Verification items for the finished model (mm, model axes). A direction names the side the tool comes from. Give positions to 0.01 mm unless a question says otherwise; leave off trailing zeros. Order: outer loops, then holes, each group sorted by start corner. A loop starts at its lowest first (then second) coordinate and runs counter-clockwise, first axis right, second up.
from build123d import *

# Parameters (mm, degrees)
SKETCH1_R           = 21.05
BOSS_EXTRUDE1_DEPTH = 10.93
SKETCH2_R           = 15.65
BOSS_EXTRUDE2_DEPTH = 0.07
SKETCH3_W           = 7.03
SKETCH3_H           = 2.225
SKETCH5_R           = 12.545
BOSS_EXTRUDE3_DEPTH = 7.14
SKETCH6_R           = 4
CUT_EXTRUDE1_DEPTH  = 19.14


with BuildPart() as part:
    # Sketch1 → Boss-Extrude1 (new body)
    with BuildSketch(Plane(origin=(0, 0, 0), x_dir=(0, 0, -1), z_dir=(1, 0, 0))):
        Circle(SKETCH1_R)
    extrude(amount=BOSS_EXTRUDE1_DEPTH)

    # Sketch2 → Boss-Extrude2 (add)
    with BuildSketch(Plane(origin=(10.93, 0, 0), x_dir=(0, 0, -1), z_dir=(1, 0, 0))):
        Circle(SKETCH2_R)
    extrude(amount=BOSS_EXTRUDE2_DEPTH)

    # Mirror1: part across plane


with BuildPart() as part_1:
    add(part.part)
    add(part.part.mirror(Plane(origin=(5.465, 0, 0), x_dir=(0, 0, 1), z_dir=(1, 0, 0))))

    # Sketch3 → Cut-Revolve1 (revolve, cut)
    with BuildSketch(Plane.XY):
        with Locations((5.465, 19.9375)):
            Rectangle(SKETCH3_W, SKETCH3_H)
    revolve(axis=Axis((0, 0, 0), (1, 0, 0)), mode=Mode.SUBTRACT)

    # Sketch5 → Boss-Extrude3 (add)
    with BuildSketch(Plane(origin=(10.93, 0, 0), x_dir=(0, 0, -1), z_dir=(1, 0, 0))):
        Circle(SKETCH5_R)
    extrude(amount=BOSS_EXTRUDE3_DEPTH)

    # Sketch6 → Cut-Extrude1 (cut, through all)
    with BuildSketch(Plane(origin=(18.07, 0, 0), x_dir=(0, 0, -1), z_dir=(1, 0, 0))):
        Circle(SKETCH6_R)
    extrude(amount=-CUT_EXTRUDE1_DEPTH, mode=Mode.SUBTRACT)


solid = part_1.part
(1) Section check D-D, the plane z = -17.5. Enter the section's corners in (x, y).
Solved:
outline: (0, -11.7) - (1.95, -11.7) - (1.95, -6.94) - (8.98, -6.94) - (8.98, -11.7) - (10.93, -11.7) - (10.93, 11.7) - (8.98, 11.7) - (8.98, 6.94) - (1.95, 6.94) - (1.95, 11.7) - (0, 11.7) - close
(2) Release check for a two-part mould opening along X. For faces 4 (the flat face through (8.98, 16, -11)), 5 (the cylindrical face through (14.49, 12.44, 1.63)), 6 (the flat face through (18.07, 3, 3)) record: pulls with the +X half, pulls with the -X half, needs draft (parallel to the pull), parting line crosses it, or undercut.
Solved:
face 4: undercut
face 5: needs draft
face 6: pulls with the +X half
(3) Set-up check for faces 1 (the flat face through (1.95, 16, -11)), 2 (the flat face through (0, 16, 0)), 3 (the flat face through (11, 5, 12)): record each of +Z, -Z, +X, -X, +Y, -Y from which the full face is reachable in a straight line by a thin tool's end or side.
Solved:
face 1: none
face 2: -X
face 3: +X
(4) Section check A-A, the plane z = 0. Enter the section's corners in (x, y) (3 decimals), then the cut area to 3 significant figures.
Solved:
outline: (-0.07, -15.65) - (0, -15.65) - (0, -21.05) - (1.95, -21.05) - (1.95, -18.825) - (8.98, -18.825) - (8.98, -21.05) - (10.93, -21.05) - (10.93, -15.65) - (11, -15.65) - (11, -12.545) - (18.07, -12.545) - (18.07, -4) - (-0.07, -4) - close; (-0.07, 4) - (18.07, 4) - (18.07, 12.545) - (11, 12.545) - (11, 15.65) - (10.93, 15.65) - (10.93, 21.05) - (8.98, 21.05) - (8.98, 18.825) - (1.95, 18.825) - (1.95, 21.05) - (0, 21.05) - (0, 15.65) - (-0.07, 15.65) - close
area: 466 mm2
(5) Section check C-C, the plane y = -10. Enter the section's corners in (x, z), then the cut area to 3 significant figures.
Solved:
outline: (-0.07, -12.04) - (0, -12.04) - (0, -18.52) - (1.95, -18.52) - (1.95, -15.95) - (8.98, -15.95) - (8.98, -18.52) - (10.93, -18.52) - (10.93, -12.04) - (11, -12.04) - (11, -7.57) - (18.07, -7.57) - (18.07, 7.57) - (11, 7.57) - (11, 12.04) - (10.93, 12.04) - (10.93, 18.52) - (8.98, 18.52) - (8.98, 15.95) - (1.95, 15.95) - (1.95, 18.52) - (0, 18.52) - (0, 12.04) - (-0.07, 12.04) - close
area: 479 mm2
(6) Scan lines: line 1 (Y direction, x = 14, z = 0) (3 decimals); line 2 (X direction, y = 17, z = -9); line 3 (Y direction, x = 15.75, z = -2). Record each from-to range of solid material in increasing order.
Solved:
line 1: y = -12.545 to -4, 4 to 12.545
line 2: x = 0 to 1.95, 8.98 to 10.93
line 3: y = -12.38 to -3.46, 3.46 to 12.38
(7) Go/stop test with flat-tipped pins: pin 1 (8 mm diameter, centred on y = 10.5, z = -14, fed in from +X); pin 2 (2 mm diameter, centred on x = 8.5, z = -13, fed in from +Y); pin 3 (10 mm diameter, centred on x = 2, z = 14, fed in from -Y); pin 4 (7 mm diameter, centred on y = 0, z = 0, fed in from +X). Record where each tip stops, or that it passes through.
Solved:
pin 1: stops at x = 11
pin 2: stops at y = 17.21
pin 3: stops at y = -19.03
pin 4: passes through
